Read the model definition and answer for the solid it produces. Units are mm, in the model's axes. A direction names the side the tool comes from. Coordinates: 2 decimals unless noted, no trailing zeros. Write each loop counter-clockwise with the first axis right and the second up, starting at its lowest first coordinate (ties: lowest second). Pieces come first, ordered by that corner, then holes. Notation, with made-up numbers: (-16, -20.5) -> (-2, -20.5) arc R18 ccw to (-2, -15.5) -> close; hole circle Ø2 at (-13, -0.5). An arc over 180 degrees is marked (long way). Use CSV: the item, a comma, the result in double quotes.
from build123d import *

# Parameters (mm, degrees)
BOSS_EXTRUDE1_DEPTH      = 9
BOSS_EXTRUDE1_DEPTH_BACK = 9
SKETCH1_W                = 12.4
SKETCH1_H                = 4.4
SKETCH1_W_2              = 10.8
SKETCH1_H_2              = 2.8
BOSS_EXTRUDE2_DEPTH      = 0.5
BOSS_EXTRUDE2_DEPTH_BACK = 0.5
BOSS_EXTRUDE3_START      = 5
BOSS_EXTRUDE3_DEPTH      = 2
CHAMFER1_SIZE            = 2
CHAMFER1_SIZE_2          = 0.76772807


with BuildPart() as part:
    # Sketch1 → Boss-Extrude1 (new, two sides: drawn at the far end of the back side and taken through both)
    with BuildSketch(Plane(origin=(0, 0, 0), x_dir=(0, 0, -1), z_dir=(1, 0, 0)).offset(-BOSS_EXTRUDE1_DEPTH_BACK)):
        Rectangle(SKETCH1_W, SKETCH1_H)
        Rectangle(SKETCH1_W_2, SKETCH1_H_2, mode=Mode.SUBTRACT)
    extrude(amount=BOSS_EXTRUDE1_DEPTH + BOSS_EXTRUDE1_DEPTH_BACK)

    # Sketch1<3> → Boss-Extrude2 (add, two sides: drawn at the far end of the back side and taken through both)
    with BuildSketch(Plane(origin=(0, 0, 0), x_dir=(0, 0, -1), z_dir=(1, 0, 0)).offset(-BOSS_EXTRUDE2_DEPTH_BACK)):
        Polygon((-5.4, 1.4), (-5.4, 0), (-4, 1.4), align=None)
        Polygon((4, 1.4), (5.4, 0), (5.4, 1.4), align=None)
        Polygon((-5.4, 0), (-5.4, -1.4), (-4, -1.4), align=None)
        Polygon((5.4, 0), (4, -1.4), (5.4, -1.4), align=None)
    extrude(amount=BOSS_EXTRUDE2_DEPTH + BOSS_EXTRUDE2_DEPTH_BACK)

    # Sketch1<4> → Boss-Extrude3 (add)
    with BuildSketch(Plane(origin=(0, 0, 0), x_dir=(0, 0, -1), z_dir=(1, 0, 0)).offset(BOSS_EXTRUDE3_START)):
        with BuildLine():
            Line((1.5, 1.4), (-1.5, 1.4))
            ThreePointArc((-1.5, 1.4), (0, 0.9), (1.5, 1.4))
        make_face()
    extrude(amount=BOSS_EXTRUDE3_DEPTH)

    # Chamfer1
    # the kernel refuses this chamfer: 2, 0.76772807 mm, written as the material it takes off along each edge
    with BuildSketch(Plane(origin=(7, 3.4, 0), x_dir=(0, 0.9120061732371908, 0.4101764741879463), z_dir=(0, 0.4101764741879463, -0.9120061732371908))) as chamfer1_piece_1_section:
        Polygon((2.5, -CHAMFER1_SIZE), (2.5 - CHAMFER1_SIZE_2, 0), (2.5, 0), align=None)
    chamfer1_piece_1 = revolve(axis=Axis((7, 3.4, 0), (1, 0, 0)), revolution_arc=311.56815777, mode=Mode.PRIVATE)
    chamfer1_piece_1 = split(chamfer1_piece_1, bisect_by=Plane(origin=(6.216344198, 1.4, 0), z_dir=(0, -1, 0)), keep=Keep.TOP, mode=Mode.PRIVATE)
    add(chamfer1_piece_1, mode=Mode.SUBTRACT)


solid = part.part
1. A cutting plane is placed at D-D (z = 3.25). Give the vertices of the cut face in (x, y).
Solutions:
outline,"(-9, -2.2) -> (9, -2.2) -> (9, -1.4) -> (-9, -1.4) -> close; (-9, 1.4) -> (9, 1.4) -> (9, 2.2) -> (-9, 2.2) -> close"
2. A cutting plane is placed at B-B (y = -0.25). Give the vertices of the cut face in (x, z), and give its area (3 significant figures).
Solutions:
outline,"(-9, -6.2) -> (9, -6.2) -> (9, -5.4) -> (0.5, -5.4) -> (0.5, -5.15) -> (-0.5, -5.15) -> (-0.5, -5.4) -> (-9, -5.4) -> close; (-9, 5.4) -> (-0.5, 5.4) -> (-0.5, 5.15) -> (0.5, 5.15) -> (0.5, 5.4) -> (9, 5.4) -> (9, 6.2) -> (-9, 6.2) -> close"
area,"29.3 mm^2"
3. Find the intervals of material crossed by line 1 along Y through (x, z) = (-2.5, 2); line 2 along Z through (x, y) = (8, 1); line 3 along X through (y, z) = (1.3, -5.25), in increasing order.
Solutions:
line 1,"y = -2.2 to -1.4, 1.4 to 2.2"
line 2,"z = -6.2 to -5.4, 5.4 to 6.2"
line 3,"x = -0.5 to 0.5"
4. A cutting plane is placed at A-A (z = -4.5). Give the vertices of the cut face in (x, y), and give its area (3 significant figures).
Solutions:
outline,"(-9, -2.2) -> (9, -2.2) -> (9, -1.4) -> (0.5, -1.4) -> (0.5, -0.9) -> (-0.5, -0.9) -> (-0.5, -1.4) -> (-9, -1.4) -> close; (-9, 1.4) -> (-0.5, 1.4) -> (-0.5, 0.9) -> (0.5, 0.9) -> (0.5, 1.4) -> (9, 1.4) -> (9, 2.2) -> (-9, 2.2) -> close"
area,"29.8 mm^2"
5. For a pull along Y with two mould halves and no side action, classify faces 1 (the flat face through (0, 0, 6.2)), 2 (the flat face through (0, -2.2, 0)), 3 (the flat face through (0, 0.7, 4.7)) as pulls with the +Y half, pulls with the -Y half, needs draft (parallel to the pull), parting line crosses it, or undercut.
Solutions:
face 1,"needs draft"
face 2,"pulls with the -Y half"
face 3,"undercut"
6. Each of these flat-tipped pins is pushed along its axis until it touches: pin 1 Ø1.5 at (y, z) = (-1, -4.5) entering from -X; pin 2 Ø0.7 at (y, z) = (-1, -4.5) entering from +X; pin 3 Ø0.7 at (y, z) = (0.5, 5) entering from -X. Where does it stop, or does it pass through?
Solutions:
pin 1,"stops at x = -9"
pin 2,"stops at x = 0.5"
pin 3,"stops at x = -0.5"
7. A tool of negligible diameter and unlimited length cuts with its end or side. For faces 4 (the flat face through (0.5, 1, -5)), 5 (the flat face through (-0.5, -1, -5)), 6 (the flat face through (0, 1.4, 0)), from which of +Z, -Z, +X, -X, +Y, -Y can it reach the whole face along a straight path? Write none if from no direction.
Solutions:
face 4,"+X"
face 5,"-X"
face 6,"none"
8. A cutting plane is placed at C-C (x = 6.5). Give the vertices of the cut face in (y, z).
Solutions:
outline,"(-2.2, -6.2) -> (2.2, -6.2) -> (2.2, 6.2) -> (-2.2, 6.2) -> close; hole (-1.4, -5.4) -> (1.4, -5.4) -> (1.4, 5.4) -> (-1.4, 5.4) -> close"
